```python
from build123d import *

# Parameters (mm, degrees)
SKETCH1_R           = 7
BOSS_EXTRUDE1_DEPTH = 3


with BuildPart() as part:
    # Sketch1 → Boss-Extrude1 (new body)
    with BuildSketch(Plane.XY):
        with BuildLine():
            ThreePointArc((-0.4997558, 7.984375), (-0.738146876, 7.96587341), (-0.975878549, 7.94025573))
            ThreePointArc((-0.975878549, 7.94025573), (-1.378121384, 7.372298248), (-1.958371564, 7.756595956))
            ThreePointArc((-1.958371564, 7.756595956), (-2.189303921, 7.694605145), (-2.418280524, 7.625740574))
            ThreePointArc((-2.418280524, 7.625740574), (-2.709312496, 6.993541721), (-3.350297333, 7.264675339))
            ThreePointArc((-3.350297333, 7.264675339), (-3.565906846, 7.161306331), (-3.778330856, 7.05153997))
            ThreePointArc((-3.778330856, 7.05153997), (-3.948241222, 6.376628518), (-4.628132745, 6.525364917))
            ThreePointArc((-4.628132745, 6.525364917), (-4.821077091, 6.384137818), (-5.009714662, 6.237207629))
            ThreePointArc((-5.009714662, 6.237207629), (-5.052717327, 5.542566879), (-5.748362647, 5.563841018))
            ThreePointArc((-5.748362647, 5.563841018), (-5.912071338, 5.389565149), (-6.070498644, 5.210474662))
            ThreePointArc((-6.070498644, 5.210474662), (-5.985129205, 4.519759773), (-6.672838954, 4.412847187))
            ThreePointArc((-6.672838954, 4.412847187), (-6.801737086, 4.211457303), (-6.924559076, 4.006305231))
            ThreePointArc((-6.924559076, 4.006305231), (-6.713724685, 3.343037668), (-7.370079733, 3.111579138))
            ThreePointArc((-7.370079733, 3.111579138), (-7.459777835, 2.889933329), (-7.542811953, 2.66570588))
            ThreePointArc((-7.542811953, 2.66570588), (-7.213692324, 2.052472426), (-7.816341286, 1.704349993))
            ThreePointArc((-7.816341286, 1.704349993), (-7.863784797, 1.469996143), (-7.904203416, 1.234329112))
            ThreePointArc((-7.904203416, 1.234329112), (-7.468006322, 0.692012696), (-7.996426712, 0.239081253))
            ThreePointArc((-7.996426712, 0.239081253), (-8, 0), (-7.996426712, -0.239081253))
            ThreePointArc((-7.996426712, -0.239081253), (-7.468006322, -0.692012696), (-7.904203416, -1.234329112))
            ThreePointArc((-7.904203416, -1.234329112), (-7.863784797, -1.469996143), (-7.816341286, -1.704349993))
            ThreePointArc((-7.816341286, -1.704349993), (-7.213692324, -2.052472426), (-7.542811953, -2.66570588))
            ThreePointArc((-7.542811953, -2.66570588), (-7.459777835, -2.889933329), (-7.370079733, -3.111579138))
            ThreePointArc((-7.370079733, -3.111579138), (-6.713724685, -3.343037668), (-6.924559076, -4.006305231))
            ThreePointArc((-6.924559076, -4.006305231), (-6.801737086, -4.211457303), (-6.672838954, -4.412847187))
            ThreePointArc((-6.672838954, -4.412847187), (-5.985129205, -4.519759773), (-6.070498644, -5.210474662))
            ThreePointArc((-6.070498644, -5.210474662), (-5.912071338, -5.389565149), (-5.748362647, -5.563841018))
            ThreePointArc((-5.748362647, -5.563841018), (-5.052717327, -5.542566879), (-5.009714662, -6.237207629))
            ThreePointArc((-5.009714662, -6.237207629), (-4.821077091, -6.384137818), (-4.628132745, -6.525364917))
            ThreePointArc((-4.628132745, -6.525364917), (-3.948241222, -6.376628518), (-3.778330856, -7.05153997))
            ThreePointArc((-3.778330856, -7.05153997), (-3.565906846, -7.161306331), (-3.350297333, -7.264675339))
            ThreePointArc((-3.350297333, -7.264675339), (-2.709312496, -6.993541721), (-2.418280524, -7.625740574))
            ThreePointArc((-2.418280524, -7.625740574), (-2.189303921, -7.694605145), (-1.958371564, -7.756595956))
            ThreePointArc((-1.958371564, -7.756595956), (-1.378121384, -7.372298248), (-0.975878549, -7.94025573))
            ThreePointArc((-0.975878549, -7.94025573), (-0.738146876, -7.96587341), (-0.4997558, -7.984375))
            ThreePointArc((-0.4997558, -7.984375), (0, -7.5), (0.4997558, -7.984375))
            ThreePointArc((0.4997558, -7.984375), (0.738146876, -7.96587341), (0.975878549, -7.94025573))
            ThreePointArc((0.975878549, -7.94025573), (1.378121384, -7.372298248), (1.958371564, -7.756595956))
            ThreePointArc((1.958371564, -7.756595956), (2.189303921, -7.694605145), (2.418280524, -7.625740574))
            ThreePointArc((2.418280524, -7.625740574), (2.709312496, -6.993541721), (3.350297333, -7.264675339))
            ThreePointArc((3.350297333, -7.264675339), (3.565906846, -7.161306331), (3.778330856, -7.05153997))
            ThreePointArc((3.778330856, -7.05153997), (3.948241222, -6.376628518), (4.628132745, -6.525364917))
            ThreePointArc((4.628132745, -6.525364917), (4.821077091, -6.384137818), (5.009714662, -6.237207629))
            ThreePointArc((5.009714662, -6.237207629), (5.052717327, -5.542566879), (5.748362647, -5.563841018))
            ThreePointArc((5.748362647, -5.563841018), (5.912071338, -5.389565149), (6.070498644, -5.210474662))
            ThreePointArc((6.070498644, -5.210474662), (5.985129205, -4.519759773), (6.672838954, -4.412847187))
            ThreePointArc((6.672838954, -4.412847187), (6.801737086, -4.211457303), (6.924559076, -4.006305231))
            ThreePointArc((6.924559076, -4.006305231), (6.713724685, -3.343037668), (7.370079733, -3.111579138))
            ThreePointArc((7.370079733, -3.111579138), (7.459777835, -2.889933329), (7.542811953, -2.66570588))
            ThreePointArc((7.542811953, -2.66570588), (7.213692324, -2.052472426), (7.816341286, -1.704349993))
            ThreePointArc((7.816341286, -1.704349993), (7.863784797, -1.469996143), (7.904203416, -1.234329112))
            ThreePointArc((7.904203416, -1.234329112), (7.468006322, -0.692012696), (7.996426712, -0.239081253))
            ThreePointArc((7.996426712, -0.239081253), (8, 0), (7.996426712, 0.239081253))
            ThreePointArc((7.996426712, 0.239081253), (7.468006322, 0.692012696), (7.904203416, 1.234329112))
            ThreePointArc((7.904203416, 1.234329112), (7.863784797, 1.469996143), (7.816341286, 1.704349993))
            ThreePointArc((7.816341286, 1.704349993), (7.213692324, 2.052472426), (7.542811953, 2.66570588))
            ThreePointArc((7.542811953, 2.66570588), (7.459777835, 2.889933329), (7.370079733, 3.111579138))
            ThreePointArc((7.370079733, 3.111579138), (6.713724685, 3.343037668), (6.924559076, 4.006305231))
            ThreePointArc((6.924559076, 4.006305231), (6.801737086, 4.211457303), (6.672838954, 4.412847187))
            ThreePointArc((6.672838954, 4.412847187), (5.985129205, 4.519759773), (6.070498644, 5.210474662))
            ThreePointArc((6.070498644, 5.210474662), (5.912071338, 5.389565149), (5.748362647, 5.563841018))
            ThreePointArc((5.748362647, 5.563841018), (5.052717327, 5.542566879), (5.009714662, 6.237207629))
            ThreePointArc((5.009714662, 6.237207629), (4.821077091, 6.384137818), (4.628132745, 6.525364917))
            ThreePointArc((4.628132745, 6.525364917), (3.948241222, 6.376628518), (3.778330856, 7.05153997))
            ThreePointArc((3.778330856, 7.05153997), (3.565906846, 7.161306331), (3.350297333, 7.264675339))
            ThreePointArc((3.350297333, 7.264675339), (2.709312496, 6.993541721), (2.418280524, 7.625740574))
            ThreePointArc((2.418280524, 7.625740574), (2.189303921, 7.694605145), (1.958371564, 7.756595956))
            ThreePointArc((1.958371564, 7.756595956), (1.378121384, 7.372298248), (0.975878549, 7.94025573))
            ThreePointArc((0.975878549, 7.94025573), (0.738146876, 7.96587341), (0.4997558, 7.984375))
            ThreePointArc((0.4997558, 7.984375), (0, 7.5), (-0.4997558, 7.984375))
        make_face()
        Circle(SKETCH1_R, mode=Mode.SUBTRACT)
    extrude(amount=BOSS_EXTRUDE1_DEPTH)


solid = part.part
```
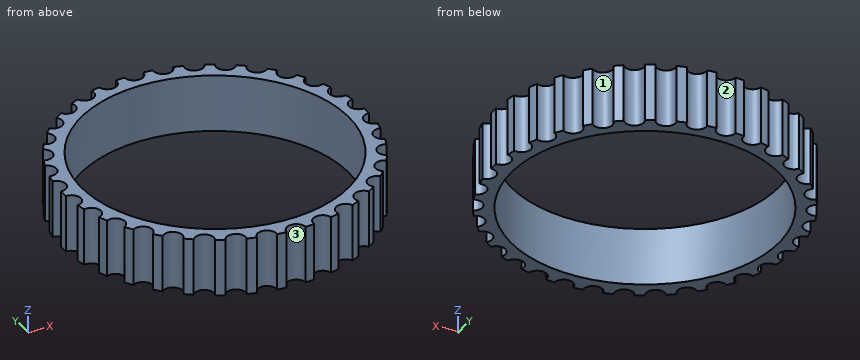
CAD build for the part. Positions are in the model's coordinates, mm. Face numbers are marked on the shaded views. Coordinates: 2 decimals unless noted, no trailing zeros. Order: outer loops, then holes, each group sorted by start corner. A loop starts at its lowest first (then second) coordinate and runs counter-clockwise, first axis right, second up. Notation, with made-up numbers: (59.25, 40) -> (71.25, 40) arc R21 cw to (71.25, 50) -> close; hole circle Ø10 at (18, -30.75). An arc over 180 degrees is marked (long way). Use one line per item in the form item = value. Start each with the question number.
1) Band-saw the part on B-B on y = 0. Give the cut face in (x, z), then the cut area to 3 significant figures.
2) Band-saw the part on A-A on x = 0. Give the cut face in (y, z), then the cut area to 3 significant figures.
3) Pull direction Y, two halves, no side cores. Call the marked faces 1, 2 and 3: +Y half, -Y half, draft (parallel to the pull), parting line (faces both ways), or undercut.
4) Drill centre lines: L1, parallel to Y at x = 0, z = 2; L2, parallel to Y at x = -0.25, z = 2.05; L3, parallel to X at y = -1.75, z = 2.35. Where is each one in solid material? Low to high. Write a range as [from, to].
5) Drop a flat-ended pin along its axis: pin 1 (1.5 mm diameter, centred on x = 5, z = 2.5, fed in from +Y). Give the stop position or say it passes through.
Entries:
q1.outline = (-8, 0) -> (-7, 0) -> (-7, 3) -> (-8, 3) -> close; (7, 0) -> (8, 0) -> (8, 3) -> (7, 3) -> close
q1.area = 6.00 mm2
q2.outline = (-7.5, 0) -> (-7, 0) -> (-7, 3) -> (-7.5, 3) -> close; (7, 0) -> (7.5, 0) -> (7.5, 3) -> (7, 3) -> close
q2.area = 3.00 mm2
q3.face_1 = undercut
q3.face_2 = +Y half
q3.face_3 = -Y half
q4.L1 = [-7.5, -7], [7, 7.5]
q4.L2 = [-7.57, -7], [7, 7.57]
q4.L3 = [-7.46, -6.78], [6.78, 7.46]
q5.pin_1 = 6.53
